Source: CAD feature listing. Evaluate the final solid. Frame: model axes, mm. A direction names the side the tool comes from. Round coordinates to 2 decimals unless told otherwise and drop trailing zeros. Write each loop counter-clockwise with the first axis right and the second up, starting at its lowest first coordinate (ties: lowest second). Pieces come first, ordered by that corner, then holes. Notation, with made-up numbers: M -17.75,55 L 8.25,55 A23 cw 8.25,70 Z; hole C -27.75,70 d8. An arc over 180 degrees is marked long. Answer in a Markdown table with one row per item.
from build123d import *

# Parameters (mm, degrees)
F1_DEPTH = 127
F3_DEPTH = 203.201


with BuildPart() as f1:
    # F0 (on Front) → F1 (new body)
    with BuildSketch(Plane.XZ):
        Polygon((101.6, -76.2), (101.6, 76.2), (50.8, 76.2), (50.8, 0), (-50.8, 0), (-50.8, 76.2), (-101.6, 76.2), (-101.6, -76.2), align=None)
    extrude(amount=F1_DEPTH)

    # F2 (on face) → F3 (cut, through all)
    with BuildSketch(Plane.YZ.offset(101.6)):
        with BuildLine():
            ThreePointArc((-127, -25.4), (-55.1579510314, 4.3579510314), (-25.4, 76.2))
            Line((-25.4, 76.2), (-127, 76.2))
            Line((-127, 76.2), (-127, -25.4))
        make_face()
    extrude(amount=-F3_DEPTH, mode=Mode.SUBTRACT)


solid = f1.part
Q1. Section C-C (z = 62). Return loops of the section in (x, y).
Solutions:
| item | result |
|---|---|
| outline | M -101.6,-26.4 L -50.8,-26.4 L -50.8,0 L -101.6,0 Z; M 50.8,-26.4 L 101.6,-26.4 L 101.6,0 L 50.8,0 Z |
Q2. Pull-direction query (X, two-part tool) for faces 1 (the flat face through (101.6, -48, -18)), 2 (the flat face through (-101.6, -48, -16)), 3 (the flat face through (1, -29, 0)), 4 (the flat face through (50.8, -16, 30)); classes: pulls with the +X half, pulls with the -X half, needs draft (parallel to the pull), parting line crosses it, or undercut.
Solutions:
| item | result |
|---|---|
| face 1 | pulls with the +X half |
| face 2 | pulls with the -X half |
| face 3 | undercut |
| face 4 | undercut |
Q3. Material intervals for probe 1 along Z at (x, y) = (36, -33); probe 2 along X at (y, z) = (-12, 38.5); probe 3 along Y at (x, z) = (-74, 9), sorted ascending.
Solutions:
| item | result |
|---|---|
| probe 1 | z = -76.2 to 0 |
| probe 2 | x = -101.6 to -50.8, 50.8 to 101.6 |
| probe 3 | y = -50.8 to 0 |
Q4. Section B-B (y = -50.5). Return loops of the section in (x, z).
Solutions:
| item | result |
|---|---|
| outline | M -101.6,-76.2 L 101.6,-76.2 L 101.6,9.34 L 50.8,9.34 L 50.8,0 L -50.8,0 L -50.8,9.34 L -101.6,9.34 Z |
Q5. Contact query for flat-ended pins moving along their axis: pin 1 Ø18 at (y, z) = (-39, 49) entering from -X; pin 2 Ø4 at (x, z) = (-48, 0.5) entering from -Y. Output: stop coordinate, or through.
Solutions:
| item | result |
|---|---|
| pin 1 | passes through |
| pin 2 | stops at y = -61.54 |
Q6. Section A-A (x = 33.5). Return loops of the section in (y, z).
Solutions:
| item | result |
|---|---|
| outline | M -127,-76.2 L 0,-76.2 L 0,0 L -59.8,0 A101.6 cw -127,-25.4 Z |
Q7. Access query for faces 5 (the flat face through (-1, 0, -16)), 6 (the flat face through (-50.8, -16, 29)). Directions: +Z, -Z, +X, -X, +Y, -Y. A direction counts if a zero-diameter tool reaches every point of the face in a straight line with its end or side. Return the directions, or none.
Solutions:
| item | result |
|---|---|
| face 5 | +Z, -Z, +X, -X, +Y |
| face 6 | +Z, +Y, -Y |
Q8. Section D-D (x = 58.5). Return loops of the section in (y, z), and give its area (3 significant figures).
Solutions:
| item | result |
|---|---|
| outline | M -127,-76.2 L 0,-76.2 L 0,76.2 L -25.4,76.2 A101.6 cw -127,-25.4 Z |
| area | 11,200 mm2 |
